Source: CAD feature listing. Evaluate the final solid. Frame: model axes, mm. Face numbers are marked on the shaded views. A direction names the side the tool comes from. Give positions to 0.01 mm unless a question says otherwise; leave off trailing zeros. Loops run counter-clockwise (first coordinate to the right, second up) from the corner with the lowest first, then second, coordinate; pieces in that order, holes last. Notation, with made-up numbers: (58.5, 52.25) -> (78.5, 52.25) arc R10 ccw to (78.5, 62.25) -> close; hole circle Ø11 at (86.5, 15.5). An arc over 180 degrees is marked (long way). Return JSON: item names as keys, results as strings. Group by question number.
(1) Access query for the marked faces 4, 5 and 6. Directions: +Z, -Z, +X, -X, +Y, -Y. A direction counts if a zero-diameter tool reaches every point of the face in a straight line with its end or side. Return the directions, or none.
(2) Cut plane B-B on y = 18.5. Return loops of the section in (x, z), then the cut area to 3 significant figures.
(3) Cut plane C-C on x = 5.25. Return loops of the section in (y, z), then the cut area to 3 significant figures.
(4) Ray query, line 1 (Z direction, x = 0, y = 12.5); line 2 (Z direction, x = 0, y = 16.25); line 3 (Y direction, x = -7.5, z = -1.75). Return the intervals inside material, ascending. Write a range as from..to.
(5) Draft query along X for the marked faces 1, 2 and 3. Return one class per face: released by +X, released by -X, zero draft, split by the parting line, or undercut.
(6) Cut plane A-A on x = 0. Return loops of the section in (y, z) (3 decimals), then the cut area to 3 significant figures.
(7) Cut plane D-D on z = 6.5. Return loops of the section in (x, y), then the cut area to 3 significant figures.
(8) Pin query (flat end, axial travel): pin 1 (5 mm diameter, centred on y = 8, z = 1, fed in from -X); pin 2 (1.6 mm diameter, centred on x = -1, z = 0.5, fed in from -Y); pin 3 (1 mm diameter, centred on y = 4.5, z = 2, fed in from +X). Return the tip coordinate at first contact, or that it passes through.
```python
from build123d import *

# Parameters (mm, degrees)
SALIENTE_EXTRUIR1_DEPTH = 13.4
CROQUIS2_R              = 6.975
CORTAR_EXTRUIR1_DEPTH   = 2.75
CROQUIS3_R              = 1.85
CORTAR_EXTRUIR2_DEPTH   = 10.65
SALIENTE_EXTRUIR2_DEPTH = 6.75
CORTAR_EXTRUIR3_START   = -6.75
CROQUIS6_R              = 1.85
CORTAR_EXTRUIR3_DEPTH   = 6.75
CROQUIS7_R              = 2.65
CORTAR_EXTRUIR4_DEPTH   = 3.5


with BuildPart() as part:
    # Croquis1 → Saliente-Extruir1 (new body)
    with BuildSketch(Plane(origin=(0, 0, 0), x_dir=(1, 0, 0), z_dir=(0, 1, 0))):
        Polygon((9.5, 0), (4.75, 8.227241336), (-4.75, 8.227241336), (-9.5, 0), (-4.75, -8.227241336), (4.75, -8.227241336), align=None)
    extrude(amount=SALIENTE_EXTRUIR1_DEPTH)

    # Croquis2 → Cortar-Extruir1 (cut)
    with BuildSketch(Plane.XZ):
        with Locations(Location((0, 0, 0), (0, 0, 270))):
            Circle(CROQUIS2_R)
    extrude(amount=-CORTAR_EXTRUIR1_DEPTH, mode=Mode.SUBTRACT)

    # Croquis3 → Cortar-Extruir2 (cut)
    with BuildSketch(Plane.XZ.offset(-2.75)):
        with Locations(Location((0, 0, 0), (0, 0, 270))):
            Circle(CROQUIS3_R)
    extrude(amount=-CORTAR_EXTRUIR2_DEPTH, mode=Mode.SUBTRACT)

    # Croquis4 → Saliente-Extruir2 (add)
    with BuildSketch(Plane(origin=(0, 13.4, 0), x_dir=(1, 0, 0), z_dir=(0, 1, 0))):
        Polygon((6.92820323, 0), (3.464101615, 6), (-3.464101615, 6), (-6.92820323, 0), (-3.464101615, -6), (3.464101615, -6), align=None)
    extrude(amount=SALIENTE_EXTRUIR2_DEPTH)

    # Croquis6 → Cortar-Extruir3 (cut)
    with BuildSketch(Plane(origin=(0, 20.15, 0), x_dir=(1, 0, 0), z_dir=(0, 1, 0)).offset(CORTAR_EXTRUIR3_START)):
        with Locations(Location((0, 0, 0), (0, 0, 90))):
            Circle(CROQUIS6_R)
    extrude(amount=CORTAR_EXTRUIR3_DEPTH, mode=Mode.SUBTRACT)

    # Croquis7 → Cortar-Extruir4 (cut)
    with BuildSketch(Plane.XZ.offset(-2.75)):
        with Locations(Location((0, 0, 0), (0, 0, 270))):
            Circle(CROQUIS7_R)
    extrude(amount=-CORTAR_EXTRUIR4_DEPTH, mode=Mode.SUBTRACT)


solid = part.part
```
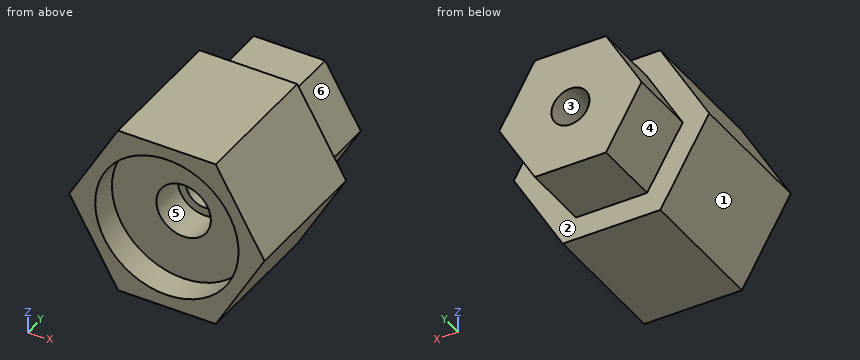
Answers:
{
 "1": {"face 4": "-Z, -X, +Y", "face 5": "-Y", "face 6": "+Z, +X, +Y"},
 "2": {"outline": "(-6.93, 0) -> (-3.46, -6) -> (3.46, -6) -> (6.93, 0) -> (3.46, 6) -> (-3.46, 6) -> close; hole circle Ø3.7 at (0, 0)", "area": "114 mm²"},
 "3": {"outline": "(0, -7.36) -> (13.4, -7.36) -> (13.4, -2.91) -> (20.15, -2.91) -> (20.15, 2.91) -> (13.4, 2.91) -> (13.4, 7.36) -> (0, 7.36) -> (0, 4.59) -> (2.75, 4.59) -> (2.75, -4.59) -> (0, -4.59) -> close", "area": "211 mm²"},
 "4": {"line 1": "-8.23..-1.85, 1.85..8.23", "line 2": "-6..-1.85, 1.85..6", "line 3": "0..13.4"},
 "5": {"face 1": "released by -X", "face 2": "zero draft", "face 3": "undercut"},
 "6": {"outline": "(0, -8.227) -> (13.4, -8.227) -> (13.4, -6) -> (20.15, -6) -> (20.15, -1.85) -> (6.25, -1.85) -> (6.25, -2.65) -> (2.75, -2.65) -> (2.75, -6.975) -> (0, -6.975) -> close; (0, 6.975) -> (2.75, 6.975) -> (2.75, 2.65) -> (6.25, 2.65) -> (6.25, 1.85) -> (20.15, 1.85) -> (20.15, 6) -> (13.4, 6) -> (13.4, 8.227) -> (0, 8.227) -> close", "area": "193 mm²"},
 "7": {"outline": "(-5.75, 0) -> (-2.53, 0) -> (-2.53, 2.75) -> (2.53, 2.75) -> (2.53, 0) -> (5.75, 0) -> (5.75, 13.4) -> (-5.75, 13.4) -> close", "area": "140 mm²"},
 "8": {"pin 1": "x = -9.5", "pin 2": "y = 6.25", "pin 3": "x = 8.63"}
}
